Geometry: final body of the model. Coordinates: model frame, mm. Face numbers are marked on the shaded views. A direction names the side the tool comes from. Give positions to 0.01 mm unless a question says otherwise; leave off trailing zeros.
```python
from build123d import *

# Parameters (mm, degrees)
SKETCH6_W               = 150
SKETCH6_H               = 40
BOSS_EXTRUDE1_DEPTH     = 130
CUT_EXTRUDE1_DEPTH      = 10
CUT_EXTRUDE2_DEPTH      = 152.410039297
CUT_EXTRUDE2_DEPTH_BACK = 152.410039297
FILLET1_R               = 20
FILLET2_R               = 5
CUT_EXTRUDE3_DEPTH      = 152.410039446
CUT_EXTRUDE3_DEPTH_BACK = 152.410039446


# Read off the part's stored shape, not the designer's step: Mirror2
with BuildPart() as part:
    # Sketch6 → Boss-Extrude1 (new body)
    with BuildSketch(Plane(origin=(0, 0, 0), x_dir=(1, 0, 0), z_dir=(0, 1, 0))):
        Rectangle(SKETCH6_W, SKETCH6_H)
    extrude(amount=BOSS_EXTRUDE1_DEPTH)

    # Sketch7 → Cut-Extrude1 (cut)
    with BuildSketch(Plane(origin=(0, 130, 0), x_dir=(1, 0, 0), z_dir=(0, 1, 0))):
        Polygon((-75, 20), (-75, 15), (-70, 15), (-70, -15), (-75, -15), (-75, -20), (75, -20), (75, -15), (70, -15), (70, 15), (75, 15), (75, 20), align=None)
    extrude(amount=-CUT_EXTRUDE1_DEPTH, mode=Mode.SUBTRACT)

    # Sketch8 → Cut-Extrude2 (cut, two sides: drawn at the far end of the back side and taken through both)
    with BuildSketch(Plane.XY.offset(-CUT_EXTRUDE2_DEPTH_BACK)):
        Polygon((-60, 120), (0, 40), (60, 120), align=None)
    extrude(amount=CUT_EXTRUDE2_DEPTH + CUT_EXTRUDE2_DEPTH_BACK, mode=Mode.SUBTRACT)

    # Fillet1
    fillet1_edges = [part.edges().sort_by_distance(p)[0] for p in [
        (0, 40, 0),
    ]]
    fillet(fillet1_edges, radius=FILLET1_R)

    # Fillet2
    fillet2_edges = [part.edges().sort_by_distance(p)[0] for p in [
        (-60, 120, 0),
        (60, 120, 0),
    ]]
    fillet(fillet2_edges, radius=FILLET2_R)

    # Sketch10 → Cut-Loft1 section 0
    with BuildSketch(Plane.XZ):
        with BuildLine():
            Line((75, 20), (75, 2))
            Line((75, 2), (0, 20))
            Line((0, 20), (75, 20))
        make_face()
    # Sketch9 → Cut-Loft1 section 1
    with BuildSketch(Plane(origin=(0, 120, 0), x_dir=(1, 0, 0), z_dir=(0, 1, 0))):
        with BuildLine():
            Line((75, -15), (75, -20))
            Line((75, -20), (70, -20))
            Line((70, -20), (75, -15))
        make_face()
    cut_loft1 = loft(mode=Mode.SUBTRACT)

    # Mirror1: Cut-Loft1 across plane
    add(cut_loft1.mirror(Plane.XY), mode=Mode.SUBTRACT)

    # Mirror2
    split(bisect_by=Plane(origin=(0, 0, 0), x_dir=(0, 0, 1), z_dir=(1, 0, 0)), keep=Keep.TOP)

    # Mirror2 2: part across plane


with BuildPart() as part_1:
    add(part.part)
    add(part.part.mirror(Plane(origin=(0, 0, 0), x_dir=(0, 0, 1), z_dir=(1, 0, 0))))

    # Sketch12 → Cut-Extrude3 (cut, two sides: drawn at the far end of the back side and taken through both)
    with BuildSketch(Plane.XY.offset(-CUT_EXTRUDE3_DEPTH_BACK)):
        Polygon((-70, 110.076825722), (-70, 63.412063573), (-42.778888747, 63.412063573), align=None)
        Polygon((-70, 51.664762149), (-70, 5), (-42.778888747, 5), align=None)
        Polygon((-68.147407502, 58.412063573), (-40.926296249, 11.747301425), (-40.926296249, 58.412063573), align=None)
        Polygon((-35.926296249, 51.664762149), (-35.926296249, 5), (-8.705184996, 5), align=None)
        Polygon((0, 43.333333333), (-28.285185422, 58.412063573), (0, 9.923174278), (28.285185422, 58.412063573), align=None)
        Polygon((40.926296249, 11.747301425), (40.926296249, 58.412063573), (68.147407502, 58.412063573), align=None)
        Polygon((8.705184996, 5), (35.926296249, 51.664762149), (35.926296249, 5), align=None)
        Polygon((70, 5), (42.778888747, 5), (70, 51.664762149), align=None)
        Polygon((70, 63.412063573), (42.778888747, 63.412063573), (70, 110.076825722), align=None)
    extrude(amount=CUT_EXTRUDE3_DEPTH + CUT_EXTRUDE3_DEPTH_BACK, mode=Mode.SUBTRACT)


solid = part_1.part
```
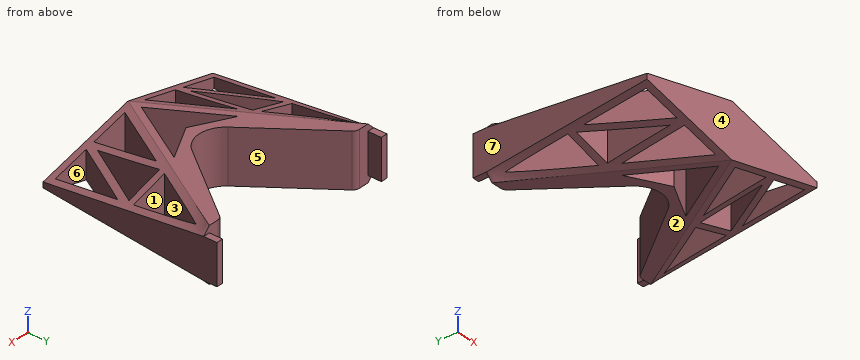
Item 1: Reachability of the marked faces 5, 6 and 7 from +Z, -Z, +X, -X, +Y, -Y: full face, straight path, thin tool, end or side. Return the list, or none.
Found:
face 5: +Z, -Z, +Y
face 6: +Z, -Z
face 7: +Z, -Z, -X, +Y, -Y
Item 2: Line query: L1, parallel to Y at x = 14, z = -1; L2, parallel to Y at x = -43, z = -1; L3, parallel to Y at x = -23.5, z = -1. Output: solid intervals per line, ascending.
Found:
L1: y = 0 to 5, 14.08 to 33.92, 50.8 to 59.05
L2: y = 0 to 5, 5.38 to 15.3, 58.41 to 63.41, 63.79 to 97.33
L3: y = 0 to 5, 30.36 to 50.21, 55.86 to 71.33
Item 3: Section A-A, the plane y = 108. State how many separate pieces and enclosed holes the cut face has, plus the area to 3 significant figures.
Found:
separate pieces: 4
enclosed holes: 0
area: 1,690 mm2
Item 4: Pull-direction query (Y, two-part tool) for the marked faces 1, 2, 3 and 4; classes: +Y half, -Y half, draft (parallel to the pull), parting line (faces both ways), or undercut.
Found:
face 1: undercut
face 2: draft
face 3: undercut
face 4: -Y half
Item 5: Pin query (flat end, axial travel): pin 1 Ø6 at (x, z) = (60, 4.5) entering from +Y; pin 2 Ø13.5 at (x, z) = (21.5, 9) entering from +Y; pin 3 Ø4 at (x, y) = (73, 124) entering from +Z. Return the tip coordinate at first contact, or that it passes through.
Found:
pin 1: stops at y = 120
pin 2: stops at y = 77.67
pin 3: stops at z = 15
